Read the model definition and answer for the solid it produces. Units are mm, in the model's axes. A direction names the side the tool comes from. Give positions to 0.01 mm unless a question says otherwise; leave off trailing zeros. Write each loop counter-clockwise with the first axis right and the second up, starting at its lowest first coordinate (ties: lowest second). Pieces come first, ordered by that corner, then holes. Notation, with made-up numbers: M 81.25,55.5 L 128.25,55.5 A28 cw 128.25,73.5 Z; hole C 36.5,62.25 d10. An arc over 180 degrees is marked long. Put each result on its own line as item: value.
from build123d import *

# Parameters (mm, degrees)
SKETCH_1_W          = 28
SKETCH_1_H          = 40
EXTRUDE_1_DEPTH     = 4
SKETCH_2_R          = 1.75
CUT_EXTRUDE_1_DEPTH = 49.989794856
SKETCH_3_W          = 46.756275812
SKETCH_3_H          = 48.920918211
CUT_EXTRUDE_2_DEPTH = 49.989794856


with BuildPart() as part:
    # 草图1 → 凸台-拉伸1 (new body)
    with BuildSketch(Plane.XY):
        with Locations((14, 20)):
            Rectangle(SKETCH_1_W, SKETCH_1_H)
    extrude(amount=EXTRUDE_1_DEPTH)

    # 草图2 → 切除-拉伸1 (cut, through all)
    with BuildSketch(Plane.XY.offset(4)):
        with Locations((7.55, 35.334562065)):
            Circle(SKETCH_2_R)
        with Locations((19.55, 35.334562065)):
            Circle(SKETCH_2_R)
        with Locations((4, 2.134562065)):
            Circle(SKETCH_2_R)
        with Locations((24, 2.134562065)):
            Circle(SKETCH_2_R)
    extrude(amount=-CUT_EXTRUDE_1_DEPTH, mode=Mode.SUBTRACT)

    # 草图3 → 切除-拉伸2 (cut, through all)
    with BuildSketch(Plane.XY.offset(4)):
        with Locations((16.027589169, 19.550398151)):
            Rectangle(SKETCH_3_W, SKETCH_3_H)
        with BuildLine():
            Line((11.5, 26.912679478), (11.5, 15.734177946))
            ThreePointArc((11.5, 15.734177946), (10.174988112, 10.759785395), (6.551083749, 7.103618696))
            Line((6.551083749, 7.103618696), (2.484674875, 4.72372984))
            ThreePointArc((2.484674875, 4.72372984), (1.424970874, 0.595333362), (5.563000373, -0.426107736))
            Line((5.563000373, -0.426107736), (8.789998756, 1.543611152))
            ThreePointArc((8.789998756, 1.543611152), (14, 3.008045147), (19.210001244, 1.543611152))
            Line((19.210001244, 1.543611152), (22.436999627, -0.426107736))
            ThreePointArc((22.436999627, -0.426107736), (26.575029126, 0.595333362), (25.515325125, 4.72372984))
            Line((25.515325125, 4.72372984), (21.448916251, 7.103618696))
            ThreePointArc((21.448916251, 7.103618696), (17.825011888, 10.759785395), (16.5, 15.734177946))
            Line((16.5, 15.734177946), (16.5, 27.172210605))
            ThreePointArc((16.5, 27.172210605), (17.147820732, 29.633619881), (18.923414249, 31.457208372))
            Line((18.923414249, 31.457208372), (21.095951451, 32.763563405))
            ThreePointArc((21.095951451, 32.763563405), (22.440760798, 36.136747835), (19.55, 38.334562065))
            Line((19.55, 38.334562065), (7.55, 38.334562065))
            ThreePointArc((7.55, 38.334562065), (4.630537584, 36.025025097), (6.206146085, 32.652388198))
            Line((6.206146085, 32.652388198), (8.739756525, 31.382969257))
            ThreePointArc((8.739756525, 31.382969257), (10.754337941, 29.539580444), (11.5, 26.912679478))
        make_face(mode=Mode.SUBTRACT)
    extrude(amount=-CUT_EXTRUDE_2_DEPTH, mode=Mode.SUBTRACT)


solid = part.part
(1) For a pull along Y with two mould halves and no side action, classify faces 1 (the face through (4, 0, 2)), 2 (the face through (4.546, 5.93, 2.028)), 3 (the face through (13, 18, 0)), 4 (the face through (23.511, 5.897, 2.028)) as +Y half, -Y half, draft (parallel to the pull), parting line (faces both ways), or undercut.
Result:
face 1: -Y half
face 2: undercut
face 3: draft
face 4: undercut
(2) Which of the six approach directions +Z, -Z, +X, -X, +Y, -Y give full straight-line access (tool end or side, diameter ignored) to faces 5 (the face through (7.455, 32.027, 2.028)), 6 (the face through (24, 0, 2)), 7 (the face through (16.5, 21, 2))?
Result:
face 5: +Z, -Z, -X
face 6: +Z, -Z, +X, -X, -Y
face 7: +Z, -Z, +X
(3) Straight lines are drawn through the part: line 1 along Y through (x, z) = (6.75, 1.25); line 2 along X through (y, z) = (34.5, 0.8); line 3 along X through (y, z) = (36, 1.4). For each, find the intervals that lie inside material, in ascending order. Write a range as from..to.
Result:
line 1: y = 0.3..7.22, 32.38..33.78, 36.89..38.23
line 2: x = 4.67..6.01, 9.09..18.01, 21.09..22.43
line 3: x = 4.62..5.93, 9.17..17.93, 21.17..22.48
(4) Section D-D on x = 14.5 is taken. Determine the outline of the cut face in (y, z), and give its area (3 significant figures).
Result:
outline: M 3,0 L 38.33,0 L 38.33,4 L 3,4 Z
area: 141 mm²
(5) Section B-B on z = 1.35 is taken. Determine the outline of the cut face in (x, y).
Result:
outline: M 1.89,0 L 6.26,0 L 8.79,1.54 A10 cw 19.21,1.54 L 21.74,0 L 26.11,0 A3 ccw 25.52,4.72 L 21.45,7.1 A10 cw 16.5,15.73 L 16.5,27.17 A5 cw 18.92,31.46 L 21.1,32.76 A3 ccw 19.55,38.33 L 7.55,38.33 A3 ccw 6.21,32.65 L 8.74,31.38 A5 cw 11.5,26.91 L 11.5,15.73 A10 cw 6.55,7.1 L 2.48,4.72 A3 ccw Z; hole C 4,2.13 d3.5; hole C 7.55,35.33 d3.5; hole C 19.55,35.33 d3.5; hole C 24,2.13 d3.5
(6) Given pin 1 Ø1 at (x, z) = (20, 1) entering from -Y; pin 2 Ø1.2 at (y, z) = (21.5, 1.5) entering from -X, each flat-ended and moving along its own axis, determine where each tip first touches the part or whether it passes through.
Result:
pin 1: stops at y = 0.76
pin 2: stops at x = 11.5
(7) Section C-C on y = 8 is taken. Determine the outline of the cut face in (x, z).
Result:
outline: M 7.84,0 L 20.16,0 L 20.16,4 L 7.84,4 Z
(8) Section A-A on x = 24 is taken. Determine the outline of the cut face in (y, z).
Result:
outline: M 0,0 L 0.38,0 L 0.38,4 L 0,4 Z; M 3.88,0 L 5.61,0 L 5.61,4 L 3.88,4 Z
